Could you check a few things on this drawing? It's one solid part, dimensions in mm from its lowest x, y, z. A direction names the side the tool comes from. Round coordinates to 2 decimals unless told otherwise and drop trailing zeros. Loops run counter-clockwise (first coordinate to the right, second up) from the corner with the lowest first, then second, coordinate; pieces in that order, holes last. Notation, with made-up numbers: (21.25, 23) -> (47.25, 23) arc R16 cw to (47.25, 33) -> close; hole circle Ø9 at (-6.75, 19). An arc over 180 degrees is marked (long way). Put each result on its own line as item: value. Start each with the question number.
1. I'm going to push flat-ended pins straight in: P1, Ø22, axis at x = 13, y = 22.5, coming from the +Z side (1 decimal); P2, Ø2, axis at y = 27.5, z = 14.5, coming from the +X side; P3, Ø2.5, axis at x = 38, y = 18.5, coming from the +Z side. Where does each tip first touch, or does it pass through?
2. Which directions (+Z, -Z, +X, -X, +Y, -Y) give clear straight access to the entire face, cutting with the end or side of a thin tool? Please do the marked faces 1, 2 and 3.
3. Imagine slicing it at A-A, the plane x = 5. Please give me the cut outline in (y, z).
4. If we mould it in two halves opening along X, with no side actions, what happens to the marked faces 4, 5, 6 and 7? For each: pulls with the +X half, pulls with the -X half, needs draft (parallel to the pull), parting line crosses it, or undercut.
5. I need wall thicknesses on line 1 (Y direction, x = 5, z = 1); line 2 (X direction, y = 23, z = 14.75); line 3 (Z direction, x = 11.5, y = 23). Which ranges of each line are inside material? Lowest first, please. Write a range as [from, to].
6. Imagine slicing it at B-B, the plane y = 22. Please give me the cut outline in (x, z), and give its area (3 significant figures).
7. Imagine slicing it at D-D, the plane x = 37.5. Please give me the cut outline in (y, z).
8. Imagine slicing it at C-C, the plane z = 10. Please give me the cut outline in (x, y), and give its area (3 significant figures).
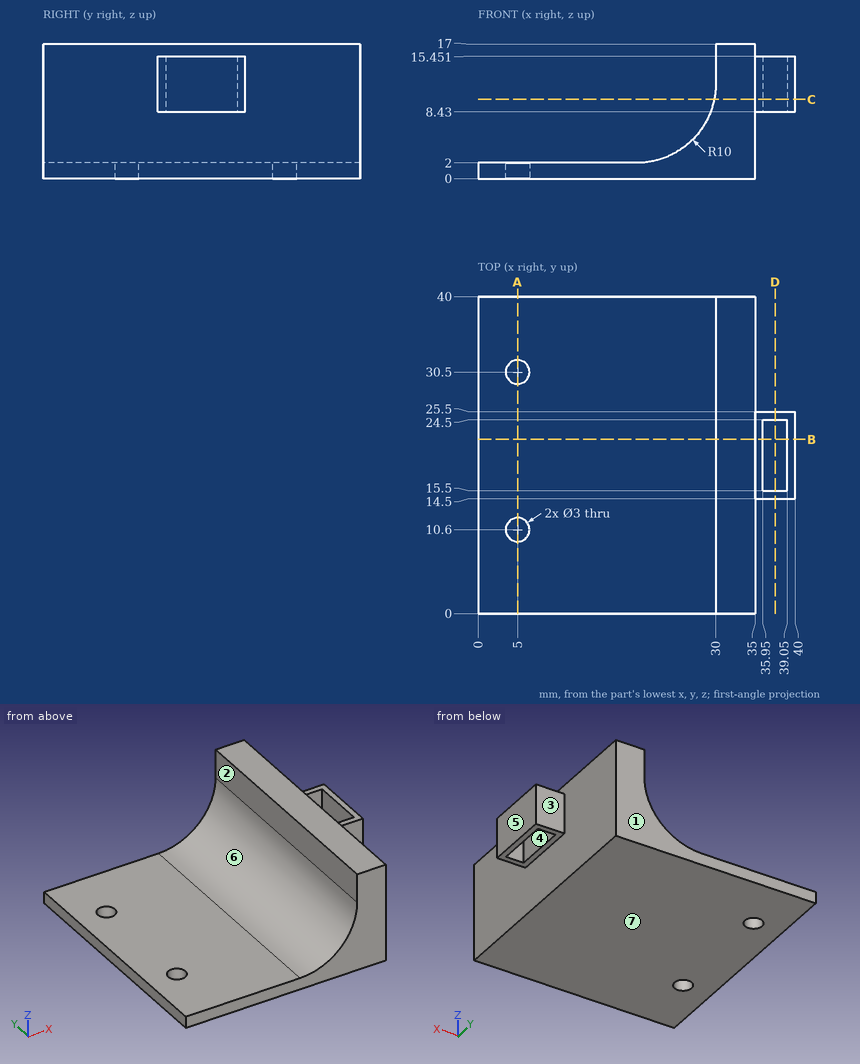
Entries:
1. P1: z = 2.8
1. P2: x = 35
1. P3: z = 15.45
2. face 1: +Z, -Z, +X, -X, +Y
2. face 2: +Z, -X, +Y, -Y
2. face 3: +Z, -Z, +X, +Y
3. outline: (0, 0) -> (9.1, 0) -> (9.1, 2) -> (0, 2) -> close; (12.1, 0) -> (29, 0) -> (29, 2) -> (12.1, 2) -> close; (32, 0) -> (40, 0) -> (40, 2) -> (32, 2) -> close
4. face 4: undercut
4. face 5: pulls with the +X half
4. face 6: pulls with the -X half
4. face 7: needs draft
5. line 1: [0, 9.1], [12.1, 29], [32, 40]
5. line 2: [30, 35.95], [39.05, 40]
5. line 3: [0, 2]
6. outline: (0, 0) -> (35, 0) -> (35, 8.43) -> (35.95, 8.43) -> (35.95, 15.45) -> (35, 15.45) -> (35, 17) -> (30, 17) -> (30, 12) arc R10 cw to (20, 2) -> (0, 2) -> close; (39.05, 8.43) -> (40, 8.43) -> (40, 15.45) -> (39.05, 15.45) -> close
6. area: 180 mm^2
7. outline: (14.5, 8.43) -> (15.5, 8.43) -> (15.5, 15.45) -> (14.5, 15.45) -> close; (24.5, 8.43) -> (25.5, 8.43) -> (25.5, 15.45) -> (24.5, 15.45) -> close
8. outline: (29.8, 0) -> (35, 0) -> (35, 14.5) -> (40, 14.5) -> (40, 25.5) -> (35, 25.5) -> (35, 40) -> (29.8, 40) -> close; hole (35.95, 15.5) -> (39.05, 15.5) -> (39.05, 24.5) -> (35.95, 24.5) -> close
8. area: 235 mm^2
